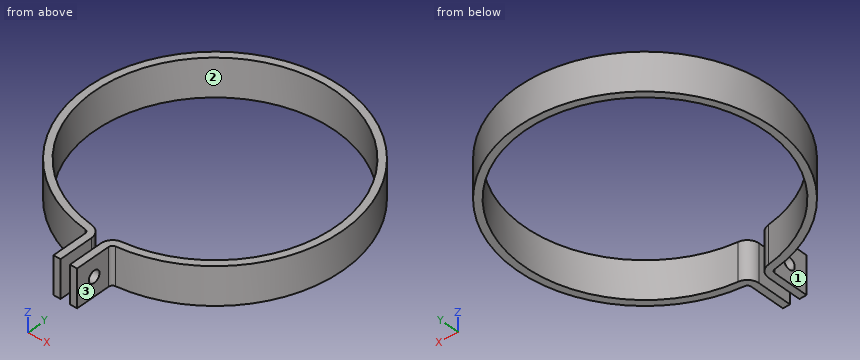
from build123d import *

# Parameters (mm, degrees)
F1_DEPTH = 50.8
F2_R     = 5.08
F3_R     = 15.875
F4_R     = 7.9375
F5_DEPTH = 187.326


with BuildPart() as f1:
    # F0 (on Top) → F1 (new body)
    with BuildSketch(Plane.XY):
        with BuildLine():
            ThreePointArc((-6.35, -161.800442), (0, 161.925), (6.35, -161.800442))
            Line((6.35, -161.800442), (6.35, -171.332367))
            Line((6.35, -171.332367), (6.35, -222.132367))
            Line((6.35, -222.132367), (15.875, -222.132367))
            Line((15.875, -222.132367), (15.875, -170.713464))
            ThreePointArc((15.875, -170.713464), (0, 171.45), (-15.875, -170.713464))
            Line((-15.875, -170.713464), (-15.875, -222.132367))
            Line((-15.875, -222.132367), (-6.35, -222.132367))
            Line((-6.35, -222.132367), (-6.35, -171.332367))
            Line((-6.35, -171.332367), (-6.35, -161.800442))
        make_face()
    extrude(amount=F1_DEPTH)

    # F2
    f2_edges = [f1.edges().sort_by_distance(p)[0] for p in [
        (-15.875, -170.713464, 25.4),
        (15.875, -170.713464, 25.4),
    ]]
    fillet(f2_edges, radius=F2_R)

    # F3
    f3_edges = [f1.edges().sort_by_distance(p)[0] for p in [
        (-6.35, -161.800442, 25.4),
        (6.35, -161.800442, 25.4),
    ]]
    fillet(f3_edges, radius=F3_R)

    # F4 (on face) → F5 (cut, through all)
    with BuildSketch(Plane(origin=(-15.875, 0, 0), x_dir=(0, -1, 0), z_dir=(-1, 0, 0))):
        with Locations((196.732367, 25.4)):
            Circle(F4_R)
    extrude(amount=-F5_DEPTH, mode=Mode.SUBTRACT)


solid = f1.part
Could you check a few things on this model? Use its own coordinates, in mm. Face numbers are marked on the shaded views. Coordinates: 2 decimals unless noted, no trailing zeros. Order: outer loops, then holes, each group sorted by start corner. A loop starts at its lowest first (then second) coordinate and runs counter-clockwise, first axis right, second up. Notation, with made-up numbers: (85.25, -30) -> (117.25, -30) arc R21 ccw to (117.25, -4) -> close; hole circle Ø5 at (-22.5, 11). An arc over 180 degrees is marked (long way). One line per item, written item: value. Start each with the question number.
1) Imagine slicing it at B-B on y = 0. List the corners of the cut face in (x, z) for me (3 decimals), plus the area to 3 significant figures.
2) I'm going to push flat-ended pins straight in: pin 1 (1.5 mm diameter, centred on y = 81, z = 39.5, fed in from +X); pin 2 (8 mm diameter, centred on y = -116.5, z = 36.5, fed in from +X); pin 3 (5 mm diameter, centred on y = -178, z = 11, fed in from -X) (3 decimals). Where does each tip first touch, or does it pass through?
3) Imagine slicing it at C-C on x = 101. List the corners of the cut face in (y, z) for me.
4) If I drill on L1, parallel to X at y = 0, z = 23 (3 decimals); L2, parallel to X at y = -204, z = 6.5 (3 decimals); L3, parallel to Y at x = 149, z = 10, over which ranges is the centre line in solid material (lowest first)? Write a range as [from, to].
5) Imagine slicing it at D-D on x = 0. List the corners of the cut face in (y, z) for me (3 decimals).
6) Imagine slicing it at A-A on z = 25.4. List the corners of the cut face in (x, y) for me (3 decimals), plus the area to 3 significant figures.
7) We'd pull the mould along X, two halves only. Please class the marked faces 1, 2 and 3: +X half, -X half, draft (parallel to the pull), parting line (faces both ways), or undercut.
Answer list:
1. outline: (-171.45, 0) -> (-161.925, 0) -> (-161.925, 50.8) -> (-171.45, 50.8) -> close; (161.925, 0) -> (171.45, 0) -> (171.45, 50.8) -> (161.925, 50.8) -> close
1. area: 968 mm2
2. pin 1: stops at x = 151.51
2. pin 2: stops at x = 129.38
2. pin 3: stops at x = -15.875
3. outline: (-138.54, 0) -> (-126.57, 0) -> (-126.57, 50.8) -> (-138.54, 50.8) -> close; (126.57, 0) -> (138.54, 0) -> (138.54, 50.8) -> (126.57, 50.8) -> close
4. L1: x = [-171.45, -161.925], [161.925, 171.45]
4. L2: x = [-15.875, -6.35], [6.35, 15.875]
4. L3: y = [-84.82, -63.39], [63.39, 84.82]
5. outline: (161.925, 0) -> (171.45, 0) -> (171.45, 50.8) -> (161.925, 50.8) -> close
6. outline: (-20.352, -170.238) arc R5.08 cw to (-15.875, -175.282) -> (-15.875, -188.795) -> (-6.35, -188.795) -> (-6.35, -176.405) arc R15.875 ccw to (-20.241, -160.655) arc R161.925 cw (long way) to (20.241, -160.655) arc R15.875 ccw to (6.35, -176.405) -> (6.35, -188.795) -> (15.875, -188.795) -> (15.875, -175.282) arc R5.08 cw to (20.352, -170.238) arc R171.45 ccw (long way) to start; (-15.875, -222.132) -> (-6.35, -222.132) -> (-6.35, -204.67) -> (-15.875, -204.67) -> close; (6.35, -222.132) -> (15.875, -222.132) -> (15.875, -204.67) -> (6.35, -204.67) -> close
6. area: 10,400 mm2
7. face 1: -X half
7. face 2: undercut
7. face 3: +X half
